Autodesk Inventor part; units mm, degrees
ref_plane "YZ Plane" through (0, 0, 0) normal (1, 0, 0) x (0, 1, 0)
ref_plane "XZ Plane" through (0, 0, 0) normal (0, 1, 0) x (-1, 0, 0)
ref_plane "XY Plane" through (0, 0, 0) normal (0, 0, 1) x (1, 0, 0)
sketch "Sketch1" plane through (0, 0, 0) normal (1, 0, 0) x (0, 1, 0)
  line L0 (0, 0) -> (139.7, 0)
  line L1 (139.7, 0) -> (139.7, -58.2676)
  line L2 (139.7, -58.2676) -> (0, -58.2676)
  line L3 (0, -58.2676) -> (0, 0)
  circle A0 centre (127, -13.2588) radius 6.35
  circle A1 centre (12.7, -45.5676) radius 4.064
  line L4 (139.7, -58.2676) -> (25.4, -58.2676)
  line L5 (25.4, -58.2676) -> (25.4, -26.5176)
  line L6 (25.4, -26.5176) -> (139.7, -26.5176)
  line L7 (139.7, -26.5176) -> (139.7, -58.2676)
  dimension "d0" = 139.7
  dimension "d2" = 12.7
  dimension "d3" = 8.128
  dimension "d5" = 114.3
  dimension "d6" = 12.7
  dimension "d7" = 12.7
  dimension "d8" = 13.2588
  dimension "d9" = 12.7
  dimension "d24" = 26.5176
  dimension "d26" = 32.3088
extrude "Extrusion1" add sketch "Sketch1" along normal blind 6.35 contours L0 L1 L6 L5 L2 L3
sketch "Sketch2" plane through (6.35, 0, 0) normal (1, 0, 0) x (0, 0, -1)
  line L0 (0, 0) -> (58.2676, 0)
  line L1 (26.5176, 139.7) -> (0, 139.7)
  line L2 (0, 139.7) -> (0, 0)
  point P0 (13.2588, 38.1)
  point P1 (13.2588, 76.2)
  dimension "d12" = 76.2
  dimension "d13" = 38.1
  dimension "d14" = 26.5176
  dimension "d15" = 13.2588
  dimension "d16" = 13.2588
hole "Hole1" at (6.35, 38.1, -13.2588) at (6.35, 76.2, -13.2588) direction (-1, 0, 0) diameter 3.81 end through all
sketch "Sketch3" plane through (0, 0, 0) normal (0, 0, 1) x (1, 0, 0)
  line L0 (0, 139.7) -> (0, 0)
  line L1 (0, 0) -> (6.35, 0)
  line L2 (6.35, 139.7) -> (6.35, 0)
  line L3 (0, 139.7) -> (6.35, 139.7)
extrude "Extrusion2" add sketch "Sketch3" along normal blind 6.35
sketch "Sketch4" plane through (6.35, 0, 0) normal (1, 0, 0) x (0, 0, -1)
  circle A0 centre (13.2588, 38.1) radius 1.905
  circle A1 centre (13.2588, 76.2) radius 1.905
  line L0 (58.2676, 25.4) -> (26.5176, 25.4)
  line L1 (26.5176, 25.4) -> (26.5176, 139.7)
  line L2 (26.5176, 139.7) -> (-6.35, 139.7)
  line L3 (-6.35, 0) -> (-6.35, 139.7)
  line L4 (58.2676, 0) -> (-6.35, 0)
  line L5 (58.2676, 0) -> (58.2676, 25.4)
  circle A2 centre (45.5676, 12.7) radius 4.064
  circle A3 centre (13.2588, 127) radius 6.35
  point P0 (0, 0)
  point P1 (-0.4699, 7.9375)
  point P2 (-0.4699, 17.4625)
  dimension "d29" = 9.525
  dimension "d30" = 7.9375
  dimension "d31" = 58.7375
  dimension "d32" = 58.7375
hole "Hole2" at (6.35, 7.9375, 0.4699) at (6.35, 17.4625, 0.4699) direction (-1, 0, 0) diameter 3.81 end through all
equation "\"d8\" = 0.5 * d24"
properties part number "PaddleCollection2.1AxleSupport" material "Nylon 6/6"
For this review, take the finished solid that the model builds, in its own axes (mm). A direction names the side the tool comes from. Give positions to 0.01 mm unless a question says otherwise; leave off trailing zeros. Order: outer loops, then holes, each group sorted by start corner. A loop starts at its lowest first (then second) coordinate and runs counter-clockwise, first axis right, second up. Notation, with made-up numbers: (82.25, 74) -> (130.25, 74) arc R18 ccw to (130.25, 106) -> close; hole circle Ø11 at (77, 42). An arc over 180 degrees is marked (long way). Write item = value, one per line.
1) We need section D-D, the plane z = -38.5. Give the boundary of the cut face in (x, y), and give its area (3 significant figures).
Findings:
outline = (0, 0) -> (6.35, 0) -> (6.35, 25.4) -> (0, 25.4) -> close
area = 161 mm^2
2) To check wall thickness, follow L1, parallel to Z at x = 4.5, y = 12.7; L2, parallel to Y at x = 3.5, z = -12.5; L3, parallel to Y at x = 0.5, z = -31.5. State the ranges of each line that lie inside material, in increasing order. Write a range as from..to.
Findings:
L1 = -58.27..-49.63, -41.5..6.35
L2 = 0..36.35, 39.85..74.45, 77.95..120.7, 133.3..139.7
L3 = 0..25.4
3) For faces 4 (the face through (3, 13, -58.268)), 5 (the face through (3, 25.4, -43)), list the 3-axis set-ups (+Z, -Z, +X, -X, +Y, -Y) from which the entire face can be reached by the end or side of a thin tool; tool diameter is ignored.
Findings:
face_4 = -Z, +X, -X, +Y, -Y
face_5 = -Z, +X, -X, +Y
4) Draft analysis for pull direction Y (two halves, no side actions). For faces 1 (the face through (3.131, 9.475, -43.095)), 2 (the face through (3, 139.7, -10)), 3 (the face through (0, 55, -19)), state which applies: pulls with the +Y half, pulls with the -Y half, needs draft (parallel to the pull), parting line crosses it, or undercut.
Findings:
face_1 = undercut
face_2 = pulls with the +Y half
face_3 = needs draft
5) We need section C-C, the plane z = -9. Give the boundary of the cut face in (x, y).
Findings:
outline = (0, 0) -> (6.35, 0) -> (6.35, 122.29) -> (0, 122.29) -> close; (0, 131.71) -> (6.35, 131.71) -> (6.35, 139.7) -> (0, 139.7) -> close
6) We need section B-B, the plane x = 3.75. Count the separate pieces of the cut face and the enclosed holes in it, and give its area (3 significant figures).
Findings:
separate_pieces = 1
enclosed_holes = 6
area = 5,170 mm^2
7) Insertion check: pin 1 (3 mm diameter, centred on x = 4.5, y = 100.5, fed in from -Z); pin 2 (10 mm diameter, centred on y = 127, z = -13.26, fed in from -X); pin 3 (3 mm diameter, centred on x = 5.5, z = -36.5, fed in from +Y). Each pin has a flat end and moves straight along its axis. Give the tip position at first contact, or say it passes through.
Findings:
pin_1 = -26.52
pin_2 = through
pin_3 = 25.4
8) We need section A-A, the plane y = 38.1. Give the boundary of the cut face in (x, z), and give its area (3 significant figures).
Findings:
outline = (0, -26.52) -> (6.35, -26.52) -> (6.35, -15.16) -> (0, -15.16) -> close; (0, -11.35) -> (6.35, -11.35) -> (6.35, 6.35) -> (0, 6.35) -> close
area = 185 mm^2
